```python
from build123d import *

# Parameters (mm, degrees)
BOSS_EXTRUDE1_DEPTH = 3
SKETCH2_R           = 2.125
CUT_EXTRUDE1_DEPTH  = 3
SKETCH3_R           = 2
CUT_EXTRUDE2_DEPTH  = 3
SKETCH4_R           = 2.125
CUT_EXTRUDE3_DEPTH  = 3
SKETCH5_W           = 470
SKETCH5_H           = 260
CUT_EXTRUDE4_DEPTH  = 3


with BuildPart() as part:
    # Sketch1 → Boss-Extrude1 (new body)
    with BuildSketch(Plane(origin=(0, 0, 0), x_dir=(1, 0, 0), z_dir=(0, 1, 0))):
        Polygon((-360, -130), (-360, 130), (-338, 130), (-338, 108), (338, 108), (338, 130), (360, 130), (360, -130), (338, -130), (338, -108), (-338, -108), (-338, -130), align=None)
    extrude(amount=BOSS_EXTRUDE1_DEPTH)

    # Sketch2 → Cut-Extrude1 (cut)
    with BuildSketch(Plane(origin=(0, 3, 0), x_dir=(1, 0, 0), z_dir=(0, 1, 0))):
        with Locations(Location((307.763857235, 49.302866975, 0), (0, 0, 270))):
            Circle(SKETCH2_R)
        with Locations(Location((282.763857235, 49.302866975, 0), (0, 0, 270))):
            Circle(SKETCH2_R)
        with Locations(Location((305.263857235, 19.302866975, 0), (0, 0, 270))):
            Circle(SKETCH2_R)
        with Locations(Location((305.263857235, -15.697133025, 0), (0, 0, 270))):
            Circle(SKETCH2_R)
        with Locations(Location((307.763857235, -45.697133025, 0), (0, 0, 270))):
            Circle(SKETCH2_R)
        with Locations(Location((282.763857235, -45.697133025, 0), (0, 0, 270))):
            Circle(SKETCH2_R)
        with Locations(Location((-287.236142765, -45.697133025, 0), (0, 0, 90))):
            Circle(SKETCH2_R)
        with Locations(Location((-312.236142765, -45.697133025, 0), (0, 0, 90))):
            Circle(SKETCH2_R)
        with Locations(Location((-309.736142765, -15.697133025, 0), (0, 0, 90))):
            Circle(SKETCH2_R)
        with Locations(Location((-309.736142765, 19.302866975, 0), (0, 0, 90))):
            Circle(SKETCH2_R)
        with Locations(Location((-287.236142765, 49.302866975, 0), (0, 0, 90))):
            Circle(SKETCH2_R)
        with Locations(Location((-312.236142765, 49.302866975, 0), (0, 0, 90))):
            Circle(SKETCH2_R)
    extrude(amount=-CUT_EXTRUDE1_DEPTH, mode=Mode.SUBTRACT)

    # Sketch3 → Cut-Extrude2 (cut)
    with BuildSketch(Plane(origin=(0, 3, 0), x_dir=(1, 0, 0), z_dir=(0, 1, 0))):
        with Locations(Location((339.440964309, 39.243831284, 0), (0, 0, 270))):
            Circle(SKETCH3_R)
        with Locations(Location((339.440964309, -36.756168716, 0), (0, 0, 90))):
            Circle(SKETCH3_R)
        with Locations(Location((-340.559035691, -36.756168716, 0), (0, 0, 270))):
            Circle(SKETCH3_R)
        with Locations(Location((-340.559035691, 39.243831284, 0), (0, 0, 90))):
            Circle(SKETCH3_R)
    extrude(amount=-CUT_EXTRUDE2_DEPTH, mode=Mode.SUBTRACT)

    # Sketch4 → Cut-Extrude3 (cut)
    with BuildSketch(Plane(origin=(0, 3, 0), x_dir=(1, 0, 0), z_dir=(0, 1, 0))):
        with Locations((66.609635331, -175.983550473)):
            Circle(SKETCH4_R)
        with Locations(Location((-179.463524521, 70.08960938, 0), (0, 0, 270))):
            Circle(SKETCH4_R)
        with Locations(Location((-15.414751286, -93.959163855, 0), (0, 0, 270))):
            Circle(SKETCH4_R)
        with Locations(Location((-97.439137904, -11.934777238, 0), (0, 0, 270))):
            Circle(SKETCH4_R)
        with Locations((77.92334383, -164.669841974)):
            Circle(SKETCH4_R)
        with Locations(Location((-4.101042787, -82.645455356, 0), (0, 0, 90))):
            Circle(SKETCH4_R)
        with Locations(Location((-86.125429405, -0.621068739, 0), (0, 0, 90))):
            Circle(SKETCH4_R)
        with Locations(Location((-168.149816022, 81.403317879, 0), (0, 0, 90))):
            Circle(SKETCH4_R)
        with Locations((-49.355876783, 200.197257118)):
            Circle(SKETCH4_R)
        with Locations((32.668509835, 118.172870501)):
            Circle(SKETCH4_R)
        with Locations(Location((114.692896452, 36.148483883, 0), (0, 0, 270))):
            Circle(SKETCH4_R)
        with Locations(Location((196.71728307, -45.875902734, 0), (0, 0, 270))):
            Circle(SKETCH4_R)
        with Locations((43.982218334, 129.486579)):
            Circle(SKETCH4_R)
        with Locations(Location((126.006604951, 47.462192382, 0), (0, 0, 90))):
            Circle(SKETCH4_R)
        with Locations((-38.042168284, 211.510965617)):
            Circle(SKETCH4_R)
        with Locations(Location((208.030991569, -34.562194235, 0), (0, 0, 90))):
            Circle(SKETCH4_R)
    extrude(amount=-CUT_EXTRUDE3_DEPTH, mode=Mode.SUBTRACT)

    # Sketch5 → Cut-Extrude4 (cut)
    with BuildSketch(Plane(origin=(0, 3, 0), x_dir=(1, 0, 0), z_dir=(0, 1, 0))):
        with Locations((125, 0)):
            Rectangle(SKETCH5_W, SKETCH5_H)
    extrude(amount=-CUT_EXTRUDE4_DEPTH, mode=Mode.SUBTRACT)


solid = part.part
```
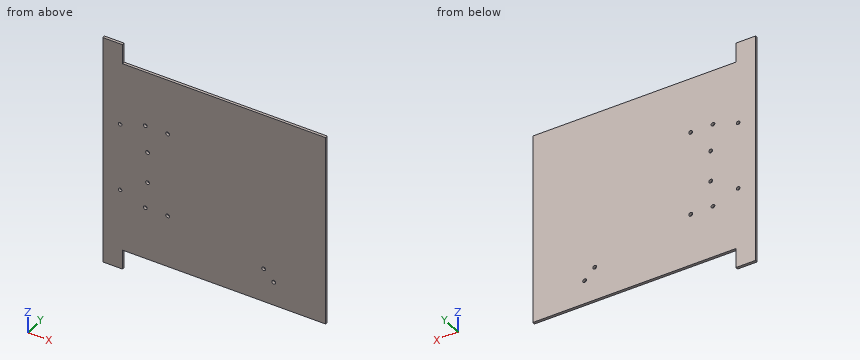
Geometry check sheet. Reference: the model listing, model coordinates, mm. Coordinates: 2 decimals unless noted, no trailing zeros. Loops run counter-clockwise (first coordinate to the right, second up) from the corner with the lowest first, then second, coordinate; pieces in that order, holes last.
Item 1: Sectioned sample at B-B, the plane z = -112. Record the boundary of the cut face in (x, y), then the cut area to 3 significant figures.
Item 2: Thickness scan on line 1 (Z direction, x = -309, y = 0.65); line 2 (Z direction, x = -209, y = 1.35); line 3 (X direction, y = 0.85, z = 37). Record the ranges inside material, lowest first.
Item 3: Sectioned sample at A-A, the plane y = 1.9. Count the separate pieces of the cut face and the enclosed holes in it, then the cut area to 3 significant figures.
Item 4: Sectioned sample at C-C, the plane x = -200. Record the boundary of the cut face in (y, z), then the cut area to 3 significant figures.
Item 5: Go/stop test with flat-tipped pins: pin 1 Ø1.5 at (y, z) = (2, -123) entering from +X; pin 2 Ø0.9 at (x, y) = (-219, 2) entering from -Z; pin 3 Ø2.5 at (x, z) = (-312.24, -49.3) entering from +Y; pin 4 Ø1.5 at (x, y) = (-254, 1.5) entering from +Z. Record where each tip stops, or that it passes through.
Check result:
1. outline: (-360, 0) - (-338, 0) - (-338, 3) - (-360, 3) - close
1. area: 66.0 mm2
2. line 1: z = -108 to -21.3, -17.31 to 13.7, 17.69 to 108
2. line 2: z = -108 to 108
2. line 3: x = -360 to -342.54, -338.57 to -110
3. separate pieces: 1
3. enclosed holes: 10
3. area: 54,800 mm2
4. outline: (0, -108) - (3, -108) - (3, 108) - (0, 108) - close
4. area: 648 mm2
5. pin 1: stops at x = -338
5. pin 2: stops at z = -108
5. pin 3: passes through
5. pin 4: stops at z = 108
